Autodesk Inventor part; units mm, degrees
ref_plane "YZ Plane" through (0, 0, 0) normal (1, 0, 0) x (0, 1, 0)
ref_plane "XZ Plane" through (0, 0, 0) normal (0, 1, 0) x (-1, 0, 0)
ref_plane "XY Plane" through (0, 0, 0) normal (0, 0, 1) x (1, 0, 0)
ref_plane "Work Plane1" through (7.7698, -13.6706, 100.9039) normal (1, 0, 0) x (0, 1, 0)
sketch "Sketch1" plane through (7.7698, -13.6706, 100.9039) normal (1, 0, 0) x (0, 1, 0)
  arc A0 (-13, -56.8488) -> (-13, -20.7888) centre (-19.0031, -38.8188) ccw
  line L0 (-26, -56.8488) -> (-13, -56.8488)
  line L1 (-13, -20.7888) -> (-26, -20.7888)
  arc A1 (-19.0031, -51.3188) -> (-19.0031, -26.3188) centre (-19.0031, -38.8188) ccw
  arc A2 (-19.0031, -56.3188) -> (-19.0031, -21.3188) centre (-19.0031, -38.8188) ccw
  arc A3 (-19.0031, -63.8188) -> (-19.0031, -13.8188) centre (-19.0031, -38.8188) ccw
  line L2 (-19.0031, -13.8188) -> (-19.0031, -63.8188)
  arc A4 (-13, -56.8488) -> (-13, -20.7888) centre (-19.0031, -38.8188) ccw
  arc A5 (-19.0031, -57.8188) -> (-19.0031, -19.8188) centre (-19.0031, -38.8188) ccw
  point P0 (13.6706, -100.9039)
  point P1 (-13.0099, -20.7888)
  point P2 (-13.0099, -56.8488)
  dimension "d0" = 12.5
  dimension "d1" = 17.5
  dimension "d2" = 25
  dimension "d3" = 19
extrude "Extrusion1" add sketch "Sketch1" along normal blind 6.5 contours A0 L1 A5 L2 A3 L0
ref_plane "Work Plane2" through (7.7698, -40.6706, 62.0852) normal (1, 0, 0) x (0, 1, 0)
sketch "Sketch2" plane through (7.7698, -40.6706, 62.0852) normal (1, 0, 0) x (0, 1, 0)
  arc A0 (14, -18.03) -> (14, 18.03) centre (7.9969, 0) ccw
  arc A1 (7.9969, -19.0031) -> (7.9969, 19.0031) centre (7.9969, 0) ccw
  arc A2 (7.9969, -17.5) -> (7.9969, 17.5) centre (7.9969, 0) ccw
  line L0 (7.9969, 19.0031) -> (7.9969, -19.0031)
  point P0 (40.6706, -62.0852)
  point P1 (14, 18.03)
  dimension "d6" = 17.5
extrude "Extrusion2" add sketch "Sketch2" against normal blind 7.5 contours A1 L0 A2 A0
sketch "Sketch3" plane through (7.7698, -40.6706, 62.0852) normal (1, 0, 0) x (0, 0, -1)
  arc A0 (17.5, 7.9969) -> (-17.5, 7.9969) centre (0, 7.9969) ccw
  arc A1 (18.03, 14) -> (-18.03, 14) centre (0, 7.9969) ccw
  arc A2 (12.5, 7.9969) -> (-12.5, 7.9969) centre (0, 7.9969) ccw
  line L0 (-17.5, 7.9969) -> (17.5, 7.9969)
  point P0 (62.0852, 40.6706)
  dimension "d9" = 12.5
extrude "Extrusion3" add sketch "Sketch3" against normal blind 18.5 contours L0 A2 A0
ref_plane "Work Plane3" through (-10.7302, -40.6706, 62.0852) normal (-1, 0, 0) x (0, 0, 1)
mirror "Mirror1" about plane through (-10.7302, -40.6706, 62.0852) normal (-1, 0, 0) of "Extrusion1", "Extrusion2", "Extrusion3"
ref_plane "Work Plane4" through (-10.7262, -56.0476, 62.0852) normal (0, 1, 0) x (-1, 0, 0)
sketch "Sketch4" plane through (-10.7262, -56.0476, 62.0852) normal (0, 1, 0) x (-1, 0, 0)
  spline S0 degree 3 poles (0, 2) (0.2512, 2) (0.5191, 1.9498) (1.0118, 1.7457) (1.2367, 1.5918) (1.5918, 1.2367) (1.7457, 1.0118) (1.9498, 0.5191) (2, 0.2512) (2, -0.2512) (1.9498, -0.5191) (1.7457, -1.0118) (1.5918, -1.2367) (1.2367, -1.5918) (1.0118, -1.7457) (0.5191, -1.9498) (0.2512, -2) (-0.2512, -2) (-0.5191, -1.9498) (-1.0118, -1.7457) (-1.2367, -1.5918) (-1.5918, -1.2367) (-1.7457, -1.0118) (-1.9498, -0.5191) (-2, -0.2512) (-2, 0.2512) (-1.9498, 0.5191) (-1.7457, 1.0118) (-1.5918, 1.2367) (-1.2367, 1.5918) (-1.0118, 1.7457) (-0.5191, 1.9498) (-0.2512, 2) (0, 2) knots 0 0 0 0 0.075352 0.075352 0.150705 0.150705 0.226057 0.226057 0.301409 0.301409 0.376761 0.376761 0.452114 0.452114 0.527466 0.527466 0.602818 0.602818 0.67817 0.67817 0.753523 0.753523 0.828875 0.828875 0.904227 0.904227 0.979579 0.979579 1.054932 1.054932 1.130284 1.130284 1.205636 1.205636 1.205636 1.205636
  point P0 (-10.7262, -62.0852)
  point P1 (0, 2)
extrude "Extrusion4" cut sketch "Sketch4" along normal through all
properties part number "BEARING TOP" material "Iron, Gray"
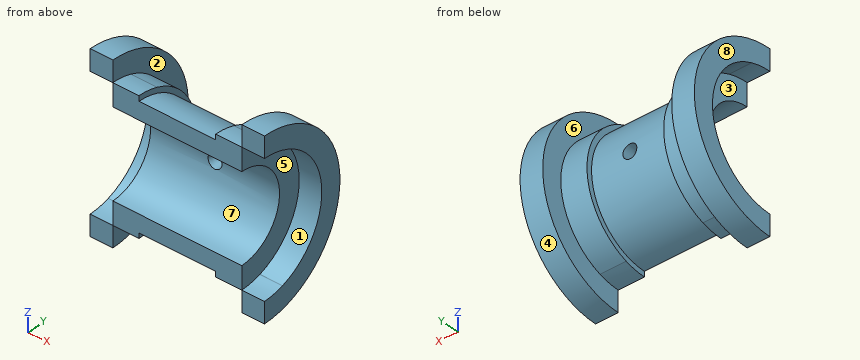
Work out the finished part from the listing and answer in its coordinate system (mm). Face numbers are marked on the shaded views. A direction names the side the tool comes from. Round coordinates to 2 decimals unless told otherwise and drop trailing zeros. Loops run counter-clockwise (first coordinate to the right, second up) from the corner with the lowest first, then second, coordinate; pieces in that order, holes last. Notation, with made-up numbers: M 59.25,13 L 98.25,13 A30 cw 98.25,48 Z; hole C 65,14.5 d9. An arc over 180 degrees is marked long. Use CSV: the item, a comma, the result in double quotes.
Q1. Section B-B, the plane z = 56 is taken. Determine the outline of the cut face in (x, y).
Determined:
outline,"M -35.73,-14.67 L -29.23,-14.67 L -29.23,-8.43 L -35.73,-8.43 Z; M -29.23,-21.75 L 7.77,-21.75 L 7.77,-14.67 L 0.27,-14.67 L 0.27,-16.27 L -21.73,-16.27 L -21.73,-14.67 L -29.23,-14.67 Z; M 7.77,-14.67 L 14.27,-14.67 L 14.27,-8.43 L 7.77,-8.43 Z"
Q2. Consider L1, parallel to X at y = -14.5, z = 52; L2, parallel to X at y = -24.5, z = 76; L3, parallel to Z at x = 11, y = -21. Determine where each line is inside the solid, lowest interval first.
Determined:
L1,"-35.73 to -29.23, 7.77 to 14.27"
L2,"-29.23 to 7.77"
L3,"39.98 to 47.09, 77.08 to 84.19"
Q3. Section A-A, the plane y = -24.25 is taken. State how many separate pieces and enclosed holes the cut face has, then the cut area to 3 significant figures.
Determined:
separate pieces,"4"
enclosed holes,"0"
area,"672 mm2"
Q4. Section C-C, the plane z = 82.5 is taken. Determine the outline of the cut face in (x, y).
Determined:
outline,"M -35.73,-32.67 L -29.23,-32.67 L -29.23,-18.24 L -35.73,-18.24 Z; M 7.77,-32.67 L 14.27,-32.67 L 14.27,-18.24 L 7.77,-18.24 Z"
Q5. A tool of negligible diameter and unlimited length cuts with its end or side. For the marked faces 1, 2, 3 and 4, from which of +Z, -Z, +X, -X, +Y, -Y can it reach the whole face along a straight path? Write none if from no direction.
Determined:
face 1,"+X, -Y"
face 2,"+Y"
face 3,"-X, -Y"
face 4,"+X, -X, +Y"
Q6. The mould has two halves that part along X. Classify the marked faces 5, 6, 7 and 8: pulls with the +X half, pulls with the -X half, needs draft (parallel to the pull), parting line crosses it, or undercut.
Determined:
face 5,"pulls with the +X half"
face 6,"undercut"
face 7,"needs draft"
face 8,"pulls with the -X half"
Q7. Each of these flat-tipped pins is pushed along its axis until it touches: pin 1 (1 mm diameter, centred on x = -17, y = -18, fed in from -Z); pin 2 (8 mm diameter, centred on x = -30.5, z = 69.5, fed in from -Y); pin 3 (10 mm diameter, centred on x = -17, z = 43, fed in from +Y). Where does it stop, or does it pass through?
Determined:
pin 1,"z = 51.82"
pin 2,"y = -27.14"
pin 3,"y = -22.29"
